from build123d import *

# Parameters (mm, degrees)
F0_R     = 27.5
F0_R_2   = 7.5
F1_DEPTH = 2
F2_R     = 27.5
F2_R_2   = 11
F3_DEPTH = 7
F4_SIZE2 = 3.49999
F4_SIZE  = 8.99999
F5_SIZE  = 1


# Not quite as in the source:
# - a fillet or chamfer is up to 0.001 mm smaller than in the source, because OpenCascade refuses the exact size


with BuildPart() as f1:
    # F0 (on Top) → F1 (new body)
    with BuildSketch(Plane.XY):
        Circle(F0_R)
        Circle(F0_R_2, mode=Mode.SUBTRACT)
    extrude(amount=F1_DEPTH)

    # F2 (on face) → F3 (join)
    with BuildSketch(Plane.XY.offset(2)):
        Circle(F2_R)
        Circle(F2_R_2, mode=Mode.SUBTRACT)
    extrude(amount=F3_DEPTH)

    # F4 (size 9 and 3.5 in the source; OpenCascade refuses exactly that, so slightly less here)
    f4_edges = [f1.edges().sort_by_distance(p)[0] for p in [
        (-27.5, 0, 0),
    ]]
    f4_side = f1.faces().sort_by_distance((-27.5, 0, 4.5))[0]
    chamfer(f4_edges, length=F4_SIZE, length2=F4_SIZE2, reference=f4_side)

    # F5
    f5_edges = [f1.edges().sort_by_distance(p)[0] for p in [
        (-11, 0, 9),
    ]]
    chamfer(f5_edges, length=F5_SIZE)


solid = f1.part
Geometry check sheet. Reference: the model listing, model coordinates, mm. A direction names the side the tool comes from. Give positions to 0.01 mm unless a question says otherwise; leave off trailing zeros. Write each loop counter-clockwise with the first axis right and the second up, starting at its lowest first coordinate (ties: lowest second). Pieces come first, ordered by that corner, then holes. Notation, with made-up numbers: (56.25, 62) - (75.25, 62) arc R10 cw to (75.25, 72) - close; hole circle Ø1 at (87.25, 37). An arc over 180 degrees is marked (long way). Put each result on its own line as item: value.
1. Thickness scan on line 1 (Y direction, x = -3.5, z = 4.25); line 2 (X direction, y = 0.5, z = 6); line 3 (Y direction, x = -4.5, z = 5.5). Record the ranges inside material, lowest first.
Ans:
line 1: y = -25.41 to -10.43, 10.43 to 25.41
line 2: x = -26.33 to -10.99, 10.99 to 26.33
line 3: y = -25.75 to -10.04, 10.04 to 25.75
2. Draft check along Y on faces 3 (the conical face through (23.054, 7.26, 0.437)), 4 (the flat face through (7.2, 2.6, 2)), 5 (the flat face through (-6, -5, 0)). Enter one of: +Y half, -Y half, draft (parallel to the pull), parting line (faces both ways), or undercut.
Ans:
face 3: parting line
face 4: undercut
face 5: draft
3. Sectioned sample at C-C, the plane z = 5.25. Enter the section's corners in (x, y), plus the area to 3 significant figures.
Ans:
outline: circle Ø52.08 at (0, 0); hole circle Ø22 at (0, 0)
area: 1,750 mm²
4. Go/stop test with flat-tipped pins: pin 1 (13.5 mm diameter, centred on x = 0, y = 0, fed in from +Z); pin 2 (1 mm diameter, centred on x = 1, z = 7, fed in from +Y); pin 3 (5 mm diameter, centred on y = -19, z = 4, fed in from +X); pin 4 (1 mm diameter, centred on x = 19, z = 5.5, fed in from -Y). Record where each tip stops, or that it passes through.
Ans:
pin 1: passes through
pin 2: stops at y = 26.9
pin 3: stops at x = 19.87
pin 4: stops at y = -18.54
5. Set-up check for faces 1 (the cylindrical face through (-2.38, -10.74, 4.96)), 2 (the cylindrical face through (-7.493, 0.33, 0.986)): record each of +Z, -Z, +X, -X, +Y, -Y from which the full face is reachable in a straight line by a thin tool's end or side.
Ans:
face 1: +Z
face 2: +Z, -Z
